Source: CAD feature listing. Evaluate the final solid. Frame: model axes, mm. A direction names the side the tool comes from. Coordinates: 2 decimals unless noted, no trailing zeros. Order: outer loops, then holes, each group sorted by start corner. A loop starts at its lowest first (then second) coordinate and runs counter-clockwise, first axis right, second up.
```python
from build123d import *

# Parameters (mm, degrees)
SKETCH1_W           = 435
SKETCH1_H           = 119.05
BOSS_EXTRUDE1_DEPTH = 19.05
SKETCH2_W           = 76.2
SKETCH2_H           = 12
CUT_EXTRUDE1_DEPTH  = 324.319973092
FILLET1_R           = 2


with BuildPart() as part:
    # Sketch1 → Boss-Extrude1 (new body)
    with BuildSketch(Plane.XY):
        with Locations((82.5, 59.525)):
            Rectangle(SKETCH1_W, SKETCH1_H)
    extrude(amount=BOSS_EXTRUDE1_DEPTH)

    # Sketch2 → Cut-Extrude1 (cut, through all)
    with BuildSketch(Plane.XY.offset(19.05)):
        Polygon((-48.8, 12), (-125, 12), (-135, 12), (-135, 0), (-125, 0), (-48.8, 0), align=None)
        with Locations((189.9, 6)):
            Rectangle(SKETCH2_W, SKETCH2_H)
    extrude(amount=-CUT_EXTRUDE1_DEPTH, mode=Mode.SUBTRACT)

    # Fillet1
    fillet1_edges = [part.edges().sort_by_distance(p)[0] for p in [
        (-48.8, 12, 9.525),
        (151.8, 12, 9.525),
        (228, 12, 9.525),
    ]]
    fillet(fillet1_edges, radius=FILLET1_R)


solid = part.part
```
1. Access query for faces 1 (the face through (79, 60, 0)), 2 (the face through (-92, 12, 10)), 3 (the face through (189, 12, 10)). Directions: +Z, -Z, +X, -X, +Y, -Y. A direction counts if a zero-diameter tool reaches every point of the face in a straight line with its end or side. Return the directions, or none.
Findings:
face 1: -Z, +X, -X, +Y, -Y
face 2: +Z, -Z, -X, -Y
face 3: +Z, -Z, -Y
2. Ray query, line 1 (X direction, y = 6, z = 14); line 2 (Y direction, x = 183.5, z = 9.25); line 3 (Y direction, x = -50, z = 17). Return the intervals inside material, ascending.
Findings:
line 1: x = -48.8 to 151.8, 228 to 300
line 2: y = 12 to 119.05
line 3: y = 11.83 to 119.05
3. Draft query along X for faces 4 (the face through (263, 0, 9)), 5 (the face through (-135, 65, 9)), 6 (the face through (228, 5, 10)). Return one class per face: released by +X, released by -X, zero draft, split by the parting line, or undercut.
Findings:
face 4: zero draft
face 5: released by -X
face 6: undercut
4. Section query A-A on z = 7.75. Return loops of the section in (x, y), plus the area to 3 significant figures.
Findings:
outline: (-135, 12) - (-50.8, 12) arc R2 cw to (-48.8, 10) - (-48.8, 0) - (151.8, 0) - (151.8, 10) arc R2 cw to (153.8, 12) - (226, 12) arc R2 cw to (228, 10) - (228, 0) - (300, 0) - (300, 119.05) - (-135, 119.05) - close
area: 49,800 mm2
5. Section query B-B on x = 163.5. Return loops of the section in (y, z).
Findings:
outline: (12, 0) - (119.05, 0) - (119.05, 19.05) - (12, 19.05) - close
6. Pin query (flat end, axial travel): P1, Ø3, axis at y = 4.5, z = 11, coming from the -X side; P2, Ø2, axis at x = -36.5, y = 76.5, coming from the -Z side; P3, Ø9.5, axis at x = 176, z = 12.5, coming from the -Y side. Return the tip coordinate at first contact, or that it passes through.
Findings:
P1: stops at x = -48.8
P2: stops at z = 0
P3: stops at y = 12
